The listing builds one solid part. Answer for the finished solid, in the listing's coordinates (mm). A direction names the side the tool comes from. Give positions to 0.01 mm unless a question says otherwise; leave off trailing zeros. Loops run counter-clockwise (first coordinate to the right, second up) from the corner with the lowest first, then second, coordinate; pieces in that order, holes last. Notation, with made-up numbers: (80.5, 60) - (91.5, 60) arc R22 cw to (91.5, 78) - close; hole circle Ø2 at (22, 35.5). An arc over 180 degrees is marked (long way). One line per item, written item: value. Start each with the question number.
from build123d import *

# Parameters (mm, degrees)
SKETCH_R        = 2
PAD_DEPTH       = 20
FILLET_R        = 4
FILLET001_R     = 4
FILLET002_R     = 4
SKETCH001_R     = 3
POCKET_DEPTH    = 11
SKETCH002_R     = 3
POCKET001_DEPTH = 13
SKETCH003_R     = 6
POCKET002_DEPTH = 3
SKETCH004_R     = 6
POCKET003_DEPTH = 5


with BuildPart() as part:
    # Sketch → Pad (new body)
    with BuildSketch(Plane.XY):
        Polygon((80, 0), (80, 12), (10, 12), (10, 40), (0, 40), (0, 0), align=None)
        with Locations((5, 30)):
            Circle(SKETCH_R, mode=Mode.SUBTRACT)
        with Locations((6, 6)):
            Circle(SKETCH_R, mode=Mode.SUBTRACT)
        with Locations((74, 6)):
            Circle(SKETCH_R, mode=Mode.SUBTRACT)
        with Locations((40, 6)):
            Circle(SKETCH_R, mode=Mode.SUBTRACT)
    extrude(amount=PAD_DEPTH)

    # Fillet
    fillet_edges = [part.edges().sort_by_distance(p)[0] for p in [
        (0, 40, 10),
    ]]
    fillet(fillet_edges, radius=FILLET_R)

    # Fillet001
    fillet001_edges = [part.edges().sort_by_distance(p)[0] for p in [
        (0, 0, 10),
    ]]
    fillet(fillet001_edges, radius=FILLET001_R)

    # Fillet002
    fillet002_edges = [part.edges().sort_by_distance(p)[0] for p in [
        (80, 0, 10),
    ]]
    fillet(fillet002_edges, radius=FILLET002_R)

    # Sketch001 → Pocket (cut)
    with BuildSketch(Plane.YZ.offset(10)):
        with Locations((20, 10)):
            Circle(SKETCH001_R)
    extrude(amount=-POCKET_DEPTH, mode=Mode.SUBTRACT)

    # Sketch002 → Pocket001 (cut)
    with BuildSketch(Plane(origin=(0, 12, 0), x_dir=(-1, 0, 0), z_dir=(0, 1, 0))):
        with Locations((-60, 10)):
            Circle(SKETCH002_R)
        with Locations((-20, 10)):
            Circle(SKETCH002_R)
    extrude(amount=-POCKET001_DEPTH, mode=Mode.SUBTRACT)

    # Sketch003 → Pocket002 (cut)
    with BuildSketch(Plane.YZ.offset(10)):
        with Locations((20, 10)):
            Circle(SKETCH003_R)
    extrude(amount=-POCKET002_DEPTH, mode=Mode.SUBTRACT)

    # Sketch004 → Pocket003 (cut)
    with BuildSketch(Plane(origin=(0, 12, 0), x_dir=(-1, 0, 0), z_dir=(0, 1, 0))):
        with Locations((-60, 10)):
            Circle(SKETCH004_R)
        with Locations((-20, 10)):
            Circle(SKETCH004_R)
    extrude(amount=-POCKET003_DEPTH, mode=Mode.SUBTRACT)


solid = part.part
1. Find the intervals of material crossed by L1, parallel to Y at x = 74, z = 9; L2, parallel to X at y = 10.5, z = 9; L3, parallel to Z at x = 20, y = 8.25, in increasing order. Write a range as [from, to].
2. A cutting plane is placed at A-A (y = 6). Determine the outline of the cut face in (x, z).
3. Flat-ended cylindrical pins translate along their axes: pin 1 (2 mm diameter, centred on x = 12, y = 14, fed in from -Z); pin 2 (6 mm diameter, centred on x = 61, z = 8, fed in from +Y); pin 3 (6 mm diameter, centred on y = 26, z = 10.5, fed in from +X); pin 4 (3.5 mm diameter, centred on y = 19, z = 7, fed in from +X). Find the tip coordinate at first contact, or state that the pin passes through.
4. A cutting plane is placed at C-C (z = 17.25). Determine the outline of the cut face in (x, y), plus the area to 3 significant figures.
5. For faces 1 (the flat face through (10, 29, 10)), 2 (the flat face through (19, 7, 13)), 3 (the flat face through (39, 0, 10)), 4 (the flat face through (7, 21, 13)), determine the directions among +Z, -Z, +X, -X, +Y, -Y from which every point of the face is accessible in a straight line to the end or side of a thin tool.
6. Determine the mould class of faces 5 (the cylindrical face through (23, 4, 10)), 6 (the cylindrical face through (75.908, 6.601, 9.86)), 7 (the flat face through (31, 11, 0)) for opening direction Z: released by +Z, released by -Z, zero draft, split by the parting line, or undercut.
7. A cutting plane is placed at D-D (y = 30). Determine the outline of the cut face in (x, z).
8. A cutting plane is placed at B-B (x = 74). Determine the outline of the cut face in (y, z), plus the area to 3 significant figures.
Results below:
1. L1: y = [0, 4], [8, 12]
1. L2: x = [0, 14.08], [25.92, 54.08], [65.92, 80]
1. L3: z = [0, 4], [16, 20]
2. outline: (0, 0) - (4, 0) - (4, 20) - (0, 20) - close; (8, 0) - (38, 0) - (38, 20) - (8, 20) - close; (42, 0) - (72, 0) - (72, 20) - (42, 20) - close; (76, 0) - (80, 0) - (80, 20) - (76, 20) - close; hole circle Ø6 at (20, 10); hole circle Ø6 at (60, 10)
3. pin 1: passes through
3. pin 2: stops at y = 7
3. pin 3: stops at x = 10
3. pin 4: stops at x = 7
4. outline: (0, 4) arc R4 ccw to (4, 0) - (76, 0) arc R4 ccw to (80, 4) - (80, 12) - (10, 12) - (10, 40) - (4, 40) arc R4 ccw to (0, 36) - close; hole circle Ø4 at (5, 30); hole circle Ø4 at (6, 6); hole circle Ø4 at (40, 6); hole circle Ø4 at (74, 6)
4. area: 1,180 mm^2
5. face 1: +Z, -Z, +X, +Y
5. face 2: +Y
5. face 3: +Z, -Z, +X, -X, -Y
5. face 4: +X
6. face 5: undercut
6. face 6: zero draft
6. face 7: released by -Z
7. outline: (0, 0) - (3, 0) - (3, 20) - (0, 20) - close; (7, 0) - (10, 0) - (10, 20) - (7, 20) - close
8. outline: (0, 0) - (4, 0) - (4, 20) - (0, 20) - close; (8, 0) - (12, 0) - (12, 20) - (8, 20) - close
8. area: 160 mm^2
